Read the model definition and answer for the solid it produces. Units are mm, in the model's axes. Face numbers are marked on the shaded views. A direction names the side the tool comes from. Coordinates: 2 decimals unless noted, no trailing zeros. Order: outer loops, then holes, each group sorted by start corner. A loop starts at its lowest first (then second) coordinate and runs counter-clockwise, first axis right, second up. Notation, with made-up numbers: (47.5, 57) - (82.5, 57) arc R12 ccw to (82.5, 62) - close; hole circle Ø9 at (54.5, 26.5). An arc over 180 degrees is marked (long way). Use one line per item in the form item = value.
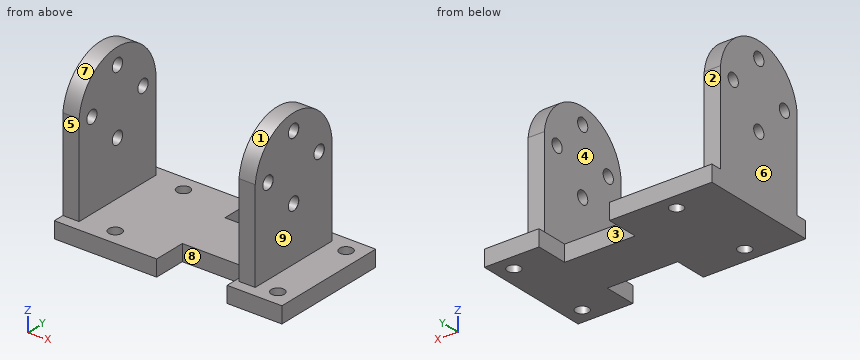
```python
from build123d import *

# Parameters (mm, degrees)
SKETCH1_W                      = 42
SKETCH1_H                      = 22
BOSS_EXTRUDE1_DEPTH            = 3
SKETCH2_W                      = 13
SKETCH2_H                      = 6
CUT_EXTRUDE1_DEPTH             = 233.19450244
SKETCH3_W                      = 13
SKETCH3_H                      = 6
CUT_EXTRUDE2_DEPTH             = 233.19450244
BOSS_EXTRUDE2_DEPTH            = 3
BOSS_EXTRUDE3_START            = -3
BOSS_EXTRUDE3_DEPTH            = 3
M2_CLEARANCE_HOLE1_D           = 2.4
M2_CLEARANCE_HOLE1_CSINK_D     = 2.45
M2_CLEARANCE_HOLE1_CSINK_ANGLE = 90
M2_CLEARANCE_HOLE2_D           = 2.4


with BuildPart() as part:
    # Sketch1 → Boss-Extrude1 (new body)
    with BuildSketch(Plane.XY.offset(163.526991532)):
        with Locations((15.20664665, 218.33461514)):
            Rectangle(SKETCH1_W, SKETCH1_H)
    extrude(amount=-BOSS_EXTRUDE1_DEPTH)

    # Sketch2 → Cut-Extrude1 (cut, through all)
    with BuildSketch(Plane(origin=(0, 0, 160.526991532), x_dir=(-1, 0, 0), z_dir=(0, 0, -1))):
        with Locations((-19.603323325, 226.33461514)):
            Rectangle(SKETCH2_W, SKETCH2_H)
    extrude(amount=-CUT_EXTRUDE1_DEPTH, mode=Mode.SUBTRACT)

    # Sketch3 → Cut-Extrude2 (cut, through all)
    with BuildSketch(Plane(origin=(0, 0, 160.526991532), x_dir=(-1, 0, 0), z_dir=(0, 0, -1))):
        with Locations((-19.603323325, 210.33461514)):
            Rectangle(SKETCH3_W, SKETCH3_H)
    extrude(amount=-CUT_EXTRUDE2_DEPTH, mode=Mode.SUBTRACT)

    # Sketch4 → Boss-Extrude2 (add)
    with BuildSketch(Plane(origin=(-5.79335335, 0, 0), x_dir=(0, -1, 0), z_dir=(-1, 0, 0))):
        with BuildLine():
            Line((-227.33461514, 180.570138914), (-227.33461514, 163.526991532))
            Line((-227.33461514, 163.526991532), (-209.33461514, 163.526991532))
            Line((-209.33461514, 163.526991532), (-209.33461514, 180.47391761))
            ThreePointArc((-209.33461514, 180.47391761), (-218.291824267, 188.52686382), (-227.33461514, 180.570138914))
        make_face()
    extrude(amount=-BOSS_EXTRUDE2_DEPTH)

    # Sketch5 → Boss-Extrude3 (add)
    with BuildSketch(Plane(origin=(29.70664665, 0, 0), x_dir=(0, 0, -1), z_dir=(1, 0, 0)).offset(BOSS_EXTRUDE3_START)):
        with BuildLine():
            Line((-180.47391761, 209.33461514), (-163.526991532, 209.33461514))
            Line((-163.526991532, 209.33461514), (-163.526991532, 227.33461514))
            Line((-163.526991532, 227.33461514), (-180.570138914, 227.33461514))
            ThreePointArc((-180.570138914, 227.33461514), (-188.52686382, 218.291824267), (-180.47391761, 209.33461514))
        make_face()
    extrude(amount=BOSS_EXTRUDE3_DEPTH)

    # M2 Clearance Hole1 (through all)
    with Locations(Plane(origin=(29.70664665, 0, 0), x_dir=(0, 0, -1), z_dir=(1, 0, 0))):
        with Locations((-179.527190494, 224.334217217), (-185.526991532, 218.334416179), (-179.527190494, 212.33461514), (-173.527389456, 218.334416179)):
            CounterSinkHole(M2_CLEARANCE_HOLE1_D / 2, M2_CLEARANCE_HOLE1_CSINK_D / 2, counter_sink_angle=M2_CLEARANCE_HOLE1_CSINK_ANGLE)

    # M2 Clearance Hole2 (through all)
    with Locations(Plane.XY.offset(163.526991532)):
        with Locations((3.103323325, 226.326974637), (3.103323325, 210.326974637), (33.103323325, 210.326974637), (33.103323325, 226.326974637)):
            Hole(M2_CLEARANCE_HOLE2_D / 2)


solid = part.part
```
(1) Given pin 1 Ø10 at (x, z) = (29.5, 172.5) entering from +Y; pin 2 Ø1.4 at (y, z) = (218.33, 173.53) entering from -X; pin 3 Ø5.5 at (y, z) = (215, 179) entering from +X; pin 4 Ø6.5 at (x, y) = (19.5, 213) entering from +Z, each flat-ended and moving along its own axis, determine where each tip first touches the part or whether it passes through.
Answer list:
pin_1 = 227.33
pin_2 = through
pin_3 = 29.71
pin_4 = 163.53
(2) Section B-B, the plane z = 175.5 is taken. Write down the section's boundary in (x, y), then the cut area to 3 significant figures.
Answer list:
outline = (-5.79, 209.33) - (-2.79, 209.33) - (-2.79, 227.33) - (-5.79, 227.33) - close; (26.71, 209.33) - (29.71, 209.33) - (29.71, 227.33) - (26.71, 227.33) - close
area = 108 mm2
(3) Section C-C, the plane y = 222.25 is taken. Write down the section's boundary in (x, z), then the cut area to 3 significant figures.
Answer list:
outline = (-5.79, 160.53) - (36.21, 160.53) - (36.21, 163.53) - (29.71, 163.53) - (29.71, 187.64) - (26.71, 187.64) - (26.71, 163.53) - (-2.79, 163.53) - (-2.79, 187.64) - (-5.79, 187.64) - close
area = 271 mm2
(4) Straight lines are drawn through the part: L1, parallel to X at y = 226.25, z = 178.5; L2, parallel to X at y = 228, z = 162; L3, parallel to Z at x = -0.5, y = 217.5. For each, find the intervals that lie inside material, in ascending order.
Answer list:
L1 = -5.79 to -2.79, 26.71 to 29.71
L2 = -5.79 to 13.1, 26.1 to 36.21
L3 = 160.53 to 163.53
(5) Section A-A, the plane y = 228 is taken. Write down the section's boundary in (x, z), then the cut area to 3 significant figures.
Answer list:
outline = (-5.79, 160.53) - (13.1, 160.53) - (13.1, 163.53) - (-5.79, 163.53) - close; (26.1, 160.53) - (36.21, 160.53) - (36.21, 163.53) - (26.1, 163.53) - close
area = 87.0 mm2
(6) Section D-D, the plane x = 23 is taken. Write down the section's boundary in (y, z).
Answer list:
outline = (213.33, 160.53) - (223.33, 160.53) - (223.33, 163.53) - (213.33, 163.53) - close
(7) Which of the six approach directions +Z, -Z, +X, -X, +Y, -Y give full straight-line access (tool end or side, diameter ignored) to the marked faces 1, 2, 3, 4 and 5?
Answer list:
face_1 = +Z, +X, -X
face_2 = +Z, +X, -X, +Y
face_3 = +Z, -Z, +Y
face_4 = +Z, +Y, -Y
face_5 = +Z, +X, -X, -Y
(8) The mould has two halves that part along X. Classify the marked faces 6, 7, 8 and 9: +X half, -X half, draft (parallel to the pull), parting line (faces both ways), or undercut.
Answer list:
face_6 = -X half
face_7 = draft
face_8 = undercut
face_9 = +X half
